Model file for the job. Use its own axes, mm. Give positions to 0.01 mm unless a question says otherwise; leave off trailing zeros. Order: outer loops, then holes, each group sorted by start corner. A loop starts at its lowest first (then second) coordinate and runs counter-clockwise, first axis right, second up. Notation, with made-up numbers: M -39,63 L -21,63 A21 ccw -21,68 Z; hole C -30.5,9 d1. An arc over 180 degrees is marked long. Return JSON: item names as keys, results as strings. Group by question number.
1. Slice it at B-B on x = -4.75. List the corners of the cut face in (y, z) (3 decimals), then the cut area to 3 significant figures.
2. Slice it at D-D on z = -5. List the corners of the cut face in (x, y), then the cut area to 3 significant figures.
3. Pin check, flat tips, straight feed: pin 1 (1.5 mm diameter, centred on x = 6, y = 2.5, fed in from -Z); pin 2 (2.5 mm diameter, centred on x = -5.6, z = -1.805, fed in from -Y). Stop position of each tip, or through.
4. Slice it at A-A on y = 3.5. List the corners of the cut face in (x, z) (3 decimals).
5. Wall check: probe 1 along X at (y, z) = (0.55, -1.5); probe 2 along X at (y, z) = (0.35, -2.5); probe 3 along Z at (x, y) = (-3.25, 0.5) (3 decimals). Give the ranges that are in metal, low to high. Write a range as [from, to].
6. Slice it at C-C on x = 5.6. List the corners of the cut face in (y, z) (3 decimals).
7. Two-plate mould, pull along Z, no slides. Class faces 1 (the face through (0, 4, -2)), 2 (the face through (6.051, 2.028, -0.374)), 3 (the face through (-6.114, 2.028, -5.683)): released by +Z, released by -Z, zero draft, split by the parting line, or undercut.
from build123d import *

# Parameters (mm, degrees)
SALIENTE_EXTRUIR1_DEPTH = 4
REDONDEO1_R             = 9
CROQUIS2_R              = 1.5
CORTAR_EXTRUIR1_DEPTH   = 15.510883067


with BuildPart() as part:
    # Croquis1 → Saliente-Extruir1 (new body)
    with BuildSketch(Plane(origin=(0, 0, 0), x_dir=(1, 0, 0), z_dir=(0, 1, 0))):
        Polygon((-6.340973223, 6.189969903), (6.340973223, 6.189969903), (12.5, 1.165), (12.5, -1.165), (-12.5, -1.165), (-12.5, 1.165), align=None)
    extrude(amount=SALIENTE_EXTRUIR1_DEPTH)

    # Redondeo1
    redondeo1_edges = [part.edges().sort_by_distance(p)[0] for p in [
        (-6.340973223, 2, -6.189969903),
        (6.340973223, 2, -6.189969903),
    ]]
    fillet(redondeo1_edges, radius=REDONDEO1_R)

    # Croquis2 → Cortar-Extruir1 (cut, through all)
    with BuildSketch(Plane(origin=(0, 4, 0), x_dir=(1, 0, 0), z_dir=(0, 1, 0))):
        with Locations(Location((-5.6, 1.805, 0), (0, 0, 270))):
            Circle(CROQUIS2_R)
        with Locations(Location((5.6, 1.805, 0), (0, 0, 270))):
            Circle(CROQUIS2_R)
    extrude(amount=-CORTAR_EXTRUIR1_DEPTH, mode=Mode.SUBTRACT)


solid = part.part
Result:
{
 "1": {"outline": "M 0,-6.044 L 4,-6.044 L 4,-3.041 L 0,-3.041 Z; M 0,-0.569 L 4,-0.569 L 4,1.165 L 0,1.165 Z", "area": "18.9 mm2"},
 "2": {"outline": "M -7.61,0 L 7.61,0 L 7.61,4 L -7.61,4 Z", "area": "60.9 mm2"},
 "3": {"pin 1": "stops at z = -5.94", "pin 2": "passes through"},
 "4": {"outline": "M -12.5,-1.165 L -8.825,-4.163 A9 ccw -3.135,-6.19 L 3.135,-6.19 A9 ccw 8.825,-4.163 L 12.5,-1.165 L 12.5,1.165 L -12.5,1.165 Z; hole C -5.6,-1.805 d3; hole C 5.6,-1.805 d3"},
 "5": {"probe 1": "x = [-12.09, -7.07], [-4.13, 4.13], [7.07, 12.09]", "probe 2": "x = [-10.86, -6.93], [-4.27, 4.27], [6.93, 10.86]", "probe 3": "z = [-6.189, 1.165]"},
 "6": {"outline": "M 0,-5.846 L 4,-5.846 L 4,-3.305 L 0,-3.305 Z; M 0,-0.305 L 4,-0.305 L 4,1.165 L 0,1.165 Z"},
 "7": {"face 1": "zero draft", "face 2": "undercut", "face 3": "released by -Z"}
}
